```python
from build123d import *

# Parameters (mm, degrees)
F2_SIZE  = 1.2
F3_R     = 1.6
F5_DEPTH = 5


# Not quite as in the source:
# - a feature names something its author has since deleted; it is built from what else it names


with BuildPart() as f1:
    # F0 (on Front) → F1 (revolve)
    with BuildSketch(Plane.XZ):
        with BuildLine():
            ThreePointArc((13.05, 6.2909673646), (14.0291561976, 5.9854143467), (14.45, 5.05))
            ThreePointArc((14.45, 5.05), (14.0838834765, 4.1661165235), (13.2, 3.8))
            Line((13.2, 3.8), (13.2, 2))
            Line((13.2, 2), (11, 2))
            Line((11, 2), (11, 0))
            Line((11, 0), (15.4, 0))
            Line((15.4, 0), (15.4, 15.4))
            Line((15.4, 15.4), (13.4, 15.4))
            Line((13.4, 15.4), (13.4, 9.05))
            Line((13.4, 9.05), (13.05, 9.05))
            Line((13.05, 9.05), (13.05, 6.2909673646))
        make_face()
    revolve(axis=Axis((0, 0, 9.4043305144), (0, 0, 1)))

    # F2
    f2_edges = [f1.edges().sort_by_distance(p)[0] for p in [
        (-11, 0, 0),
        (-15.4, 0, 0),
        (-15.4, 0, 15.4),
    ]]
    chamfer(f2_edges, length=F2_SIZE)

    # F3
    f3_edges = [f1.edges().sort_by_distance(p)[0] for p in [
        (-13.05, 0, 6.290967),
        (-13.2, 0, 3.8),
    ]]
    fillet(f3_edges, radius=F3_R)

    # F4 (on face) → F5 (join)
    with BuildSketch(Plane.XY.offset(9.05)):
        with BuildLine():
            ThreePointArc((0.1999944308, 13.3985074627), (0.1999986077, 13.3992537261), (0.2, 13.4))
            ThreePointArc((0.2, 13.4), (-0.0007462739, 13.5999986077), (-0.1999944308, 13.3985074627))
            ThreePointArc((-0.1999944308, 13.3985074627), (0, 13.4), (0.1999944308, 13.3985074627))
        make_face()
        with BuildLine():
            ThreePointArc((0.1999944308, 13.3985074627), (0, 13.4), (-0.1999944308, 13.3985074627))
            ThreePointArc((-0.1999944308, 13.3985074627), (0, 13.2), (0.1999944308, 13.3985074627))
        make_face()
        with BuildLine():
            ThreePointArc((-11.4047404107, -6.7), (-11.5040948148, -6.527169262), (-11.7034450509, -6.5260534737))
            ThreePointArc((-11.7034450509, -6.5260534737), (-11.6047404107, -6.7), (-11.5034506201, -6.872453989))
            ThreePointArc((-11.5034506201, -6.872453989), (-11.4311633988, -6.7993530117), (-11.4047404107, -6.7))
        make_face()
        with BuildLine():
            ThreePointArc((11.5034506201, -6.872453989), (11.6047404107, -6.7), (11.7034450509, -6.5260534737))
            ThreePointArc((11.7034450509, -6.5260534737), (11.43153533, -6.6), (11.5034506201, -6.872453989))
        make_face()
    extrude(amount=F5_DEPTH)


solid = f1.part
```
Geometry: final body of the model. Coordinates: model frame, mm. A direction names the side the tool comes from. Round coordinates to 2 decimals unless told otherwise and drop trailing zeros. Loops run counter-clockwise (first coordinate to the right, second up) from the corner with the lowest first, then second, coordinate; pieces in that order, holes last. Notation, with made-up numbers: (17, 14.5) -> (32, 14.5) arc R31 cw to (32, 42.5) -> close; hole circle Ø7 at (66.5, -21). An arc over 180 degrees is marked (long way). Use one line per item in the form item = value. Start each with the question number.
1) Access query for faces 1 (the cylindrical face through (-2.38, -10.74, 1.59)), 2 (the cylindrical face through (-13.387, 0.589, 12.181)). Directions: +Z, -Z, +X, -X, +Y, -Y. A direction counts if a zero-diameter tool reaches every point of the face in a straight line with its end or side. Return the directions, or none.
2) First-contact query: P1, Ø10, axis at x = -5, y = 7.5, coming from the +Z side; P2, Ø6, axis at x = -7.5, z = 3.5, coming from the -Y side; P3, Ø1, axis at y = -7.5, z = 10.5, coming from the -X side; P4, Ø1, axis at y = -11, z = 8.5, coming from the -X side. Flat tips, straight axial feed; report the tip coordinate or a pass-through.
3) Line query: L1, parallel to Y at x = 0, z = 2.5; L2, parallel to Y at x = 0, z = 8.3; L3, parallel to Z at x = -12, y = -4. Output: solid intervals per line, ascending.
4) Draft query along Z for faces 3 (the cylindrical face through (-1.718, 13.088, 2.341)), 4 (the cylindrical face through (-3.338, -15.034, 7.791)), 5 (the flat face through (-6, 11, 0)), 6 (the flat face through (11.8, 6, 9.05)). Return one class per face: released by +Z, released by -Z, zero draft, split by the parting line, or undercut.
5) Section A-A on z = 10. Output: boundary loops of the cut face in (x, y).
6) Section B-B on z = 4.5. Output: boundary loops of the cut face in (x, y) (1 decimal), then the cut area to 3 significant figures.
Response:
q1.face_1 = +Z, -Z
q1.face_2 = +Z
q2.P1 = 15.4
q2.P2 = -14.73
q2.P3 = -13.72
q2.P4 = -11.27
q3.L1 = -15.4 to -13.2, 13.2 to 15.4
q3.L2 = -15.4 to -13.05, 13.05 to 15.4
q3.L3 = 0 to 2
q4.face_3 = undercut
q4.face_4 = zero draft
q4.face_5 = released by -Z
q4.face_6 = released by +Z
q5.outline = circle Ø30.8 at (0, 0); hole (-11.7, -6.53) arc R0.2 cw to (-11.5, -6.87) arc R13.4 ccw to (11.5, -6.87) arc R0.2 cw to (11.7, -6.53) arc R13.4 ccw to (0.2, 13.4) arc R0.2 cw to (-0.2, 13.4) arc R13.4 ccw to start
q6.outline = circle Ø30.8 at (0, 0); hole circle Ø28.6 at (0, 0)
q6.area = 101 mm^2
